Could you check a few things on this model? Use its own coordinates, in mm. Give positions to 0.01 mm unless a question says otherwise; leave off trailing zeros. Loops run counter-clockwise (first coordinate to the right, second up) from the corner with the lowest first, then second, coordinate; pieces in that order, holes last.
1. Imagine slicing it at C-C (x = 133). List the corners of the cut face in (y, z) for me (3 decimals), plus the area to 3 significant figures.
2. Imagine slicing it at B-B (x = 252). List the corners of the cut face in (y, z) for me (3 decimals).
3. Imagine slicing it at A-A (z = 2). Count the separate pieces of the cut face and the enclosed holes in it, plus the area to 3 significant figures.
4. I need wall thicknesses on line 1 along X through (y, z) = (10, 1.25); line 2 along Y through (x, z) = (110, 2.95); line 3 along Y through (x, z) = (325, 1.25). Which ranges of each line are inside material? Lowest first, please.
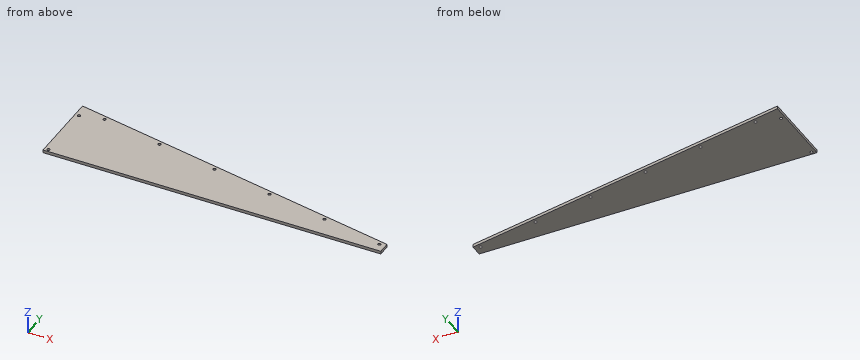
Autodesk Inventor part; units mm, degrees
ref_plane "YZ Plane" through (0, 0, 0) normal (1, 0, 0) x (0, 1, 0)
ref_plane "XZ Plane" through (0, 0, 0) normal (0, 1, 0) x (-1, 0, 0)
ref_plane "XY Plane" through (0, 0, 0) normal (0, 0, 1) x (1, 0, 0)
sketch "Sketch1" plane through (0, 0, 0) normal (0, 0, 1) x (1, 0, 0)
  line L0 (0, 0) -> (0, 88.9)
  line L1 (0, 88.9) -> (366.2791, 19.3046)
  line L2 (467.8791, 0) -> (366.2791, 0) construction
  line L3 (366.2791, 0) -> (366.2791, 19.3046)
  line L4 (366.2791, 19.3046) -> (467.8791, 0) construction
  line L5 (366.2791, 0) -> (0, 0)
  line L6 (0, 6.35) -> (366.2791, 6.35)
  circle A0 centre (4.3656, 73.025) radius 1.5875
  circle A1 centre (4.3656, 9.525) radius 1.5875
  line L7 (11.9063, 82.55) -> (-3.9687, 82.55) construction
  line L8 (11.9063, 82.55) -> (11.9063, 0) construction
  line L9 (-3.9687, 0) -> (11.9063, 0) construction
  line L10 (-3.9687, 82.55) -> (-3.9687, 0) construction
  circle A2 centre (293.5291, 28.6839) radius 1.5875
  circle A3 centre (161.2752, 53.8129) radius 1.5875
  circle A4 centre (29.0214, 78.942) radius 1.5875
  circle A5 centre (95.1483, 66.3775) radius 1.5875
  circle A6 centre (227.4022, 41.2484) radius 1.5875
  circle A7 centre (359.656, 16.1193) radius 1.5875
  line L11 (21.2196, 88.9079) -> (18.2563, 73.3119) construction
  line L12 (21.2196, 88.9079) -> (370.5693, 22.5292) construction
  line L13 (367.606, 6.9333) -> (370.5693, 22.5292) construction
  line L14 (18.2563, 73.3119) -> (367.606, 6.9333) construction
  dimension "d0" = 88.9
  dimension "d1" = 476.25
  dimension "d5" = 101.6
  dimension "d6" = 6.35
extrude "Extrusion1" add sketch "Sketch1" along normal blind 3.175 contours L0 L1 L3 L6
properties part number "Hopper Back Wedge Side" material "Polycarbonate, Clear"
Derived:
1. outline: (6.35, 0) - (63.629, 0) - (63.629, 3.175) - (6.35, 3.175) - close
1. area: 182 mm2
2. outline: (6.35, 0) - (41.018, 0) - (41.018, 3.175) - (6.35, 3.175) - close
3. separate pieces: 1
3. enclosed holes: 8
3. area: 17,400 mm2
4. line 1: x = 0 to 2.85, 5.88 to 366.28
4. line 2: y = 6.35 to 68
4. line 3: y = 6.35 to 27.15
